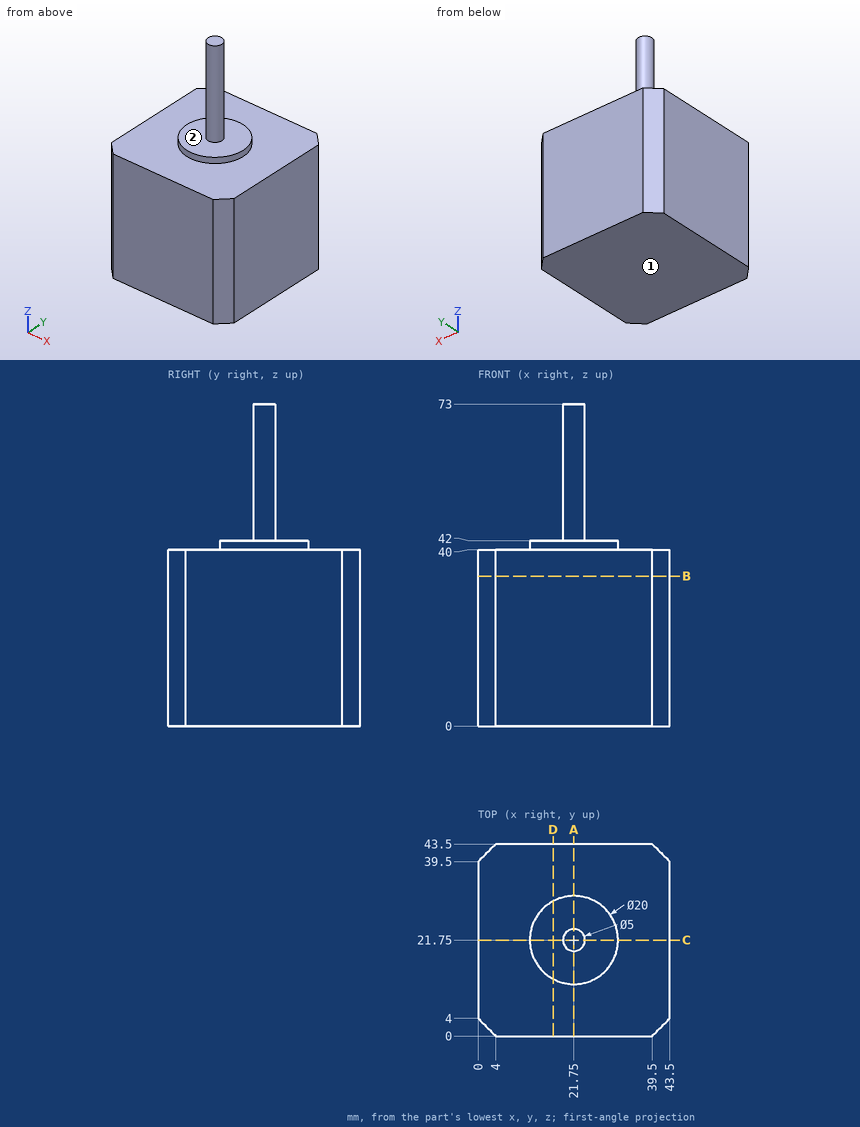
Here's the drawing with two shaded views (mm, measured from the low corner). I have some questions. A direction names the side the tool comes from. Give positions to 0.01 mm unless a question says otherwise; leave off trailing zeros. Order: outer loops, then holes, each group sorted by start corner. A loop starts at its lowest first (then second) coordinate and runs counter-clockwise, first axis right, second up. Notation, with made-up numbers: M -23.75,-1.75 L 17.25,-1.75 A32 ccw 17.25,25.25 Z; hole C -10,4.5 d10. An arc over 180 degrees is marked long. One line per item, written item: value.
1) I want a section at A-A, the plane x = 21.75. List the corners of the cut face in (y, z) for me.
Answer sheet:
outline: M 0,0 L 43.5,0 L 43.5,40 L 31.75,40 L 31.75,42 L 24.25,42 L 24.25,73 L 19.25,73 L 19.25,42 L 11.75,42 L 11.75,40 L 0,40 Z
2) Please list where these lines run through material, in increasing order: line 1 along Z through (x, y) = (39, 34.5); line 2 along Z through (x, y) = (19, 25); line 3 along Y through (x, z) = (3.5, 18).
Answer sheet:
line 1: z = 0 to 40
line 2: z = 0 to 42
line 3: y = 0.5 to 43
3) I want a section at B-B, the plane z = 34. List the corners of the cut face in (x, y) for me, plus the area to 3 significant figures.
Answer sheet:
outline: M 0,4 L 4,0 L 39.5,0 L 43.5,4 L 43.5,39.5 L 39.5,43.5 L 4,43.5 L 0,39.5 Z
area: 1,860 mm^2
4) On a 3-axis mill with a long thin cutter (end or side, diameter ignored), from which of +Z, -Z, +X, -X, +Y, -Y can I reach the whole of each face in a straight line? I mean the marked faces 1 and 2. Say none if no direction works.
Answer sheet:
face 1: -Z, +X, -X, +Y, -Y
face 2: +Z
5) For P1, Ø1.5, axis at x = 20, y = 30.5, coming from the +Z side; P2, Ø6, axis at x = 16, z = 57, coming from the -Y side; P3, Ø12, axis at x = 11.5, y = 37.5, coming from the +Z side; P4, Ø5, axis at y = 26.5, z = 59, coming from the -X side, each with a flat end and sliding along its axis, tell me the tip position at first contact or that it passes through.
Answer sheet:
P1: stops at z = 42
P2: passes through
P3: stops at z = 40
P4: stops at x = 20.66
6) I want a section at D-D, the plane x = 17. List the corners of the cut face in (y, z) for me, plus the area to 3 significant figures.
Answer sheet:
outline: M 0,0 L 43.5,0 L 43.5,40 L 30.55,40 L 30.55,42 L 12.95,42 L 12.95,40 L 0,40 Z
area: 1,780 mm^2
